CAD build for the part. Positions are in the model's coordinates, mm. Face numbers are marked on the shaded views. A direction names the side the tool comes from. Give positions to 0.01 mm unless a question says otherwise; leave off trailing zeros. Loops run counter-clockwise (first coordinate to the right, second up) from the corner with the lowest first, then second, coordinate; pieces in that order, holes last.
Item 1: Mould opens along X. For the marked faces 1, 2 and 3 say: released by +X, released by -X, zero draft, split by the parting line, or undercut.
Item 2: Saw through at B-B on y = -5. Give the cut face in (x, z), plus the area to 3 significant figures.
Item 3: Probe probe 1 along X at (y, z) = (3.5, 0); probe 2 along X at (y, z) = (8, 0); probe 3 along X at (y, z) = (-11, -2.75). List the from-to ranges inside material, lowest first.
Item 4: Drop flat-ended pins along their axis: P1, Ø6.5, axis at x = 4.45, z = 0, coming from the +Y side; P2, Ø6, axis at x = -4.45, z = 0, coming from the -Y side; P3, Ø3, axis at x = -5.5, y = 8.5, coming from the -Z side; P4, Ø1, axis at x = -1, y = 8, coming from the +Z side. Give the stop position or say it passes through.
Item 5: Saw through at C-C on x = -2.5. Give the cut face in (y, z).
Item 6: Saw through at D-D on x = 1.25. Give the cut face in (y, z), plus the area to 3 significant figures.
Item 7: Which spindle directions (+Z, -Z, +X, -X, +Y, -Y) get a long thin tool onto all of the face, cutting with end or side? Do the marked faces 4, 5 and 6. Say none if no direction does.
Item 8: Saw through at A-A on z = 0. Give the number of separate pieces and of enclosed holes in the cut face, plus the area to 3 significant figures.
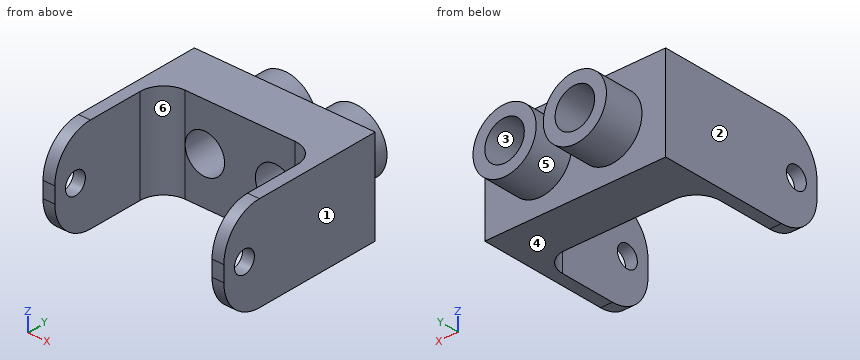
from build123d import *

# Parameters (mm, degrees)
BOSS_EXTRUDE1_OUTLINE_W = 22.9
BOSS_EXTRUDE1_OUTLINE_H = 12
BOSS_EXTRUDE1_DEPTH     = 6.3
SKETCH2_R               = 4
BOSS_EXTRUDE2_DEPTH     = 5
SKETCH3_R               = 2.5
CUT_EXTRUDE1_DEPTH      = 11.3
SKETCH4_W               = 1.5
SKETCH4_H               = 12
BOSS_EXTRUDE3_DEPTH     = 15
FILLET1_R               = 3
CUT_EXTRUDE2_REACH      = 30.025
SKETCH5_R               = 1.4
FILLET2_R               = 5


# Read off the part's stored shape, not the designer's step: Boss-Extrude1
with BuildPart() as part:
    # Boss-Extrude1 outline → Boss-Extrude1 (new body)
    with BuildSketch(Plane(origin=(0, 0, 0), x_dir=(1, 0, 0), z_dir=(0, 1, 0))):
        Rectangle(BOSS_EXTRUDE1_OUTLINE_W, BOSS_EXTRUDE1_OUTLINE_H)
    extrude(amount=BOSS_EXTRUDE1_DEPTH)

    # Sketch2 → Boss-Extrude2 (add)
    with BuildSketch(Plane(origin=(0, 6.3, 0), x_dir=(1, 0, 0), z_dir=(0, 1, 0))):
        with Locations(Location((-4.45, 0, 0), (0, 0, 90))):
            Circle(SKETCH2_R)
        with Locations(Location((4.45, 0, 0), (0, 0, 90))):
            Circle(SKETCH2_R)
    extrude(amount=BOSS_EXTRUDE2_DEPTH)

    # Sketch3 → Cut-Extrude1 (cut)
    with BuildSketch(Plane(origin=(0, 11.3, 0), x_dir=(1, 0, 0), z_dir=(0, 1, 0))):
        with Locations(Location((4.45, 0, 0), (0, 0, 270))):
            Circle(SKETCH3_R)
        with Locations(Location((-4.45, 0, 0), (0, 0, 270))):
            Circle(SKETCH3_R)
    extrude(amount=-CUT_EXTRUDE1_DEPTH, mode=Mode.SUBTRACT)

    # Sketch4 → Boss-Extrude3 (add)
    with BuildSketch(Plane.XZ):
        with Locations((-10.7, 0)):
            Rectangle(SKETCH4_W, SKETCH4_H)
        with Locations((10.7, 0)):
            Rectangle(SKETCH4_W, SKETCH4_H)
    extrude(amount=BOSS_EXTRUDE3_DEPTH)

    # Fillet1
    fillet1_edges = [part.edges().sort_by_distance(p)[0] for p in [
        (9.95, 0, 0),
        (-9.95, 0, 0),
    ]]
    fillet(fillet1_edges, radius=FILLET1_R - 0.0001)  # a hair under: the kernel refuses the full size

    # Cut-Extrude2: up to this face of the body (flat: up to its plane)
    cut_extrude2_end = Plane(part.part.faces().sort_by_distance((11.45, -4.35, 0))[0])
    # Sketch5 → Cut-Extrude2 (cut, up to the picked face)
    with BuildSketch(Plane.ZY.offset(11.45), mode=Mode.PRIVATE) as cut_extrude2_sk1:
        with Locations((0, -12.1)):
            Circle(SKETCH5_R)
    cut_extrude2_tool1 = split(extrude(cut_extrude2_sk1.sketch, amount=-CUT_EXTRUDE2_REACH, mode=Mode.PRIVATE), bisect_by=cut_extrude2_end, keep=Keep.BOTH, mode=Mode.PRIVATE)
    add(cut_extrude2_tool1.solids().sort_by(Axis((-11.45, -12.1, 0), (1, 0, 0)))[0], mode=Mode.SUBTRACT)

    # Fillet2
    fillet2_edges = [part.edges().sort_by_distance(p)[0] for p in [
        (-10.7, -15, -6),
        (-10.7, -15, 6),
        (10.7, -15, -6),
        (10.7, -15, 6),
    ]]
    fillet(fillet2_edges, radius=FILLET2_R)


solid = part.part
Results below:
1. face 1: released by +X
1. face 2: released by -X
1. face 3: undercut
2. outline: (-11.45, -6) - (-9.95, -6) - (-9.95, 6) - (-11.45, 6) - close; (9.95, -6) - (11.45, -6) - (11.45, 6) - (9.95, 6) - close
2. area: 36.0 mm2
3. probe 1: x = -11.45 to -6.95, -1.95 to 1.95, 6.95 to 11.45
3. probe 2: x = -8.45 to -6.95, -1.95 to -0.45, 0.45 to 1.95, 6.95 to 8.45
3. probe 3: x = -11.45 to -9.95, 9.95 to 11.45
4. P1: stops at y = 11.3
4. P2: stops at y = -0.04
4. P3: stops at z = -4
4. P4: stops at z = 2.7
5. outline: (0, -6) - (6.3, -6) - (6.3, -3.49) - (11.3, -3.49) - (11.3, -1.56) - (0, -1.56) - close; (0, 1.56) - (11.3, 1.56) - (11.3, 3.49) - (6.3, 3.49) - (6.3, 6) - (0, 6) - close
6. outline: (0, -6) - (6.3, -6) - (6.3, -2.4) - (11.3, -2.4) - (11.3, 2.4) - (6.3, 2.4) - (6.3, 6) - (0, 6) - close
6. area: 99.6 mm2
7. face 4: -Z, +X, -X, +Y, -Y
7. face 5: +Y
7. face 6: +Z, -Z, -Y
8. separate pieces: 5
8. enclosed holes: 0
8. area: 152 mm2
